from build123d import *

# Parameters (mm, degrees)
SKETCH1_W               = 50
SKETCH1_H               = 30
BOSS_EXTRUDE1_DEPTH     = 5
CUT_EXTRUDE3_DEPTH      = 1
CUT_EXTRUDE3_DEPTH_BACK = 31
CUT_EXTRUDE4_DEPTH      = 26
CUT_EXTRUDE4_DEPTH_BACK = 26


with BuildPart() as part:
    # Sketch1 → Boss-Extrude1 (new body)
    with BuildSketch(Plane.XY):
        Rectangle(SKETCH1_W, SKETCH1_H)
    extrude(amount=BOSS_EXTRUDE1_DEPTH)

    # Sketch4 → Cut-Extrude3 (cut, two sides)
    with BuildSketch(Plane(origin=(0, 15, 0), x_dir=(1, 0, 0), z_dir=(0, 1, 0))) as cut_extrude3_sk:
        Polygon((-25, -5), (-20, 0), (-25, 0), align=None)
        Polygon((25, -5), (20, 0), (25, 0), align=None)
    extrude(amount=CUT_EXTRUDE3_DEPTH, mode=Mode.SUBTRACT)
    extrude(cut_extrude3_sk.sketch, amount=-CUT_EXTRUDE3_DEPTH_BACK, mode=Mode.SUBTRACT)

    # Sketch5 → Cut-Extrude4 (cut, two sides)
    with BuildSketch(Plane(origin=(0, 0, 0), x_dir=(0, 0, -1), z_dir=(1, 0, 0))) as cut_extrude4_sk:
        Polygon((-5, -15), (0, -10), (0, -15), align=None)
    extrude(amount=CUT_EXTRUDE4_DEPTH, mode=Mode.SUBTRACT)
    extrude(cut_extrude4_sk.sketch, amount=-CUT_EXTRUDE4_DEPTH_BACK, mode=Mode.SUBTRACT)


solid = part.part
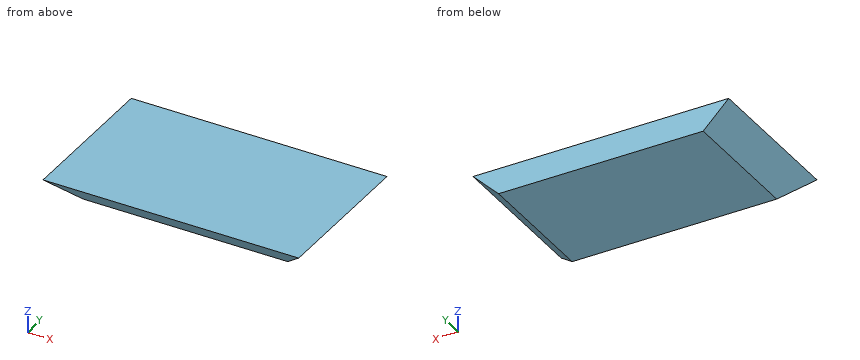
For this review, take the finished solid that the model builds, in its own axes (mm). Give positions to 0.01 mm unless a question says otherwise; leave off trailing zeros. Write each loop counter-clockwise with the first axis right and the second up, starting at its lowest first coordinate (ties: lowest second). Pieces come first, ordered by that corner, then holes. Notation, with made-up numbers: (-1.5, 40) -> (11.5, 40) arc R30 cw to (11.5, 74) -> close; hole circle Ø5 at (56, 78). An arc over 180 degrees is marked (long way). Use CSV: the item, a comma, the result in double quotes.
Q1. Take a section at B-B, the plane y = -6. Write out the cut boundary in (x, z).
Conclusion:
outline,"(-25, 5) -> (-20, 0) -> (20, 0) -> (25, 5) -> close"
Q2. To check wall thickness, follow probe 1 along Y at (x, z) = (4, 4.5); probe 2 along Y at (x, z) = (-20, 0.7); probe 3 along X at (y, z) = (3, 0.7). State the ranges of each line that lie inside material, in increasing order. Write a range as [from, to].
Conclusion:
probe 1,"[-14.5, 15]"
probe 2,"[-10.7, 15]"
probe 3,"[-20.7, 20.7]"
Q3. For P1, Ø1.5, axis at y = 11, z = 4, coming from the +X side; P2, Ø2, axis at y = -1.5, z = 3.5, coming from the -X side; P3, Ø1.5, axis at x = 5.5, z = 3.5, coming from the -Y side, all flat-tipped, find the tip position at first contact; note any pin that passes through.
Conclusion:
P1,"x = 24.75"
P2,"x = -24.5"
P3,"y = -14.25"
Q4. Take a section at A-A, the plane x = 10. Write out the cut boundary in (y, z), then the cut area to 4 significant figures.
Conclusion:
outline,"(-15, 5) -> (-10, 0) -> (15, 0) -> (15, 5) -> close"
area,"137.5 mm2"
